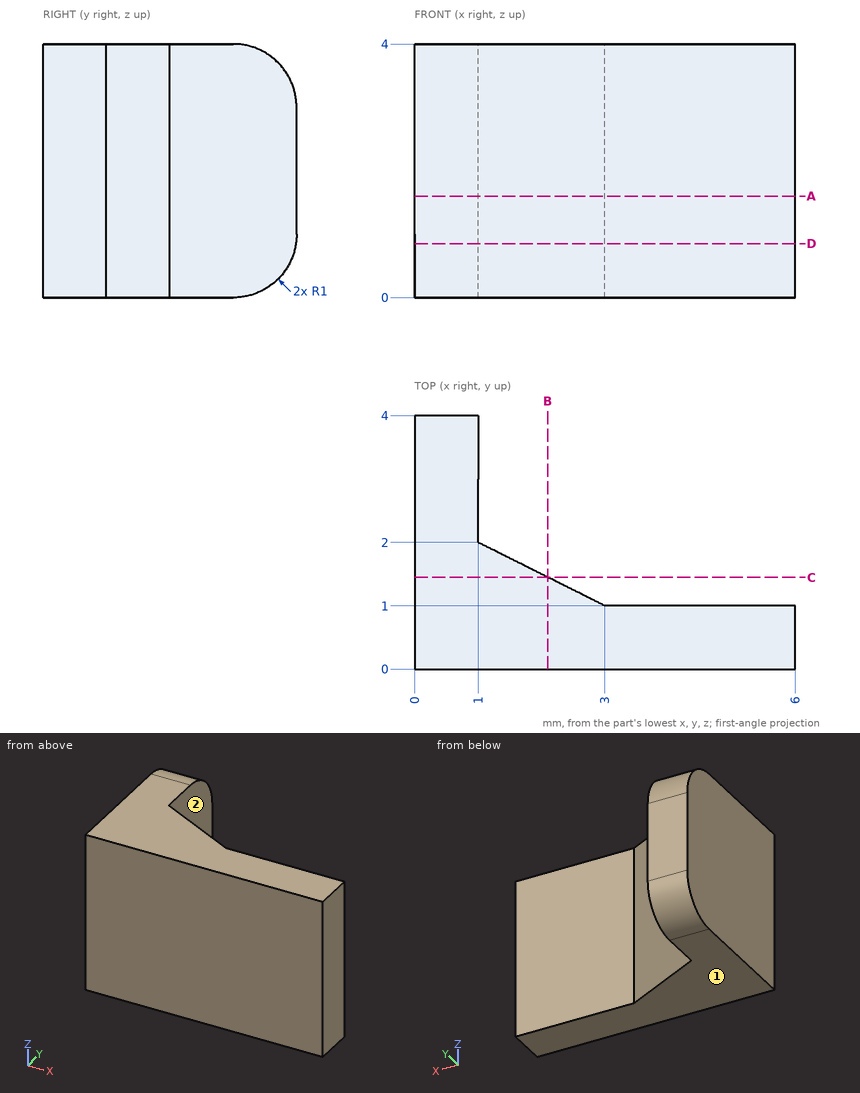
The drawing under review shows one solid part. Ordinate dimensions are in mm from its lowest x, y, z. A direction names the side the tool comes from. Round coordinates to 2 decimals unless told otherwise and drop trailing zeros. Write each loop counter-clockwise with the first axis right and the second up, starting at its lowest first coordinate (ties: lowest second). Pieces come first, ordered by that corner, then holes.
(1) We need section D-D on z = 0.85. Give the boundary of the cut face in (x, y), and give its area (3 significant figures).
(2) Insertion check: pin 1 (2 mm diameter, centred on y = 3.5, z = 3, fed in from +X); pin 2 (1.5 mm diameter, centred on y = 2, z = 2.5, fed in from +X). Each pin has a flat end and moves straight along its axis. Give the tip position at first contact, or say it passes through.
(3) We need section C-C on y = 1.45. Give the boundary of the cut face in (x, z).
(4) We need section A-A on z = 1.6. Give the boundary of the cut face in (x, y).
(5) Machinability: for the marked faces 1 and 2, which of the approach directions +Z, -Z, +X, -X, +Y, -Y give a long, thin tool a straight path to every point of the face, cutting with its end or side? Answer none if there is none.
(6) Wall thickness on L1, parallel to X at y = 3.65, z = 2.4; L2, parallel to X at y = 1.5, z = 2.65: over which ranges is each line inside the solid? List them lowest first.
(7) We need section B-B on x = 2.1. Give the boundary of the cut face in (y, z), and give its area (3 significant figures).
Findings below:
1. outline: (0, 0) - (6, 0) - (6, 1) - (3, 1) - (1, 2) - (1, 3.99) - (0, 3.99) - close
1. area: 9.99 mm2
2. pin 1: stops at x = 1
2. pin 2: stops at x = 2.5
3. outline: (0, 0) - (2.1, 0) - (2.1, 4) - (0, 4) - close
4. outline: (0, 0) - (6, 0) - (6, 1) - (3, 1) - (1, 2) - (1, 4) - (0, 4) - close
5. face 1: -Z, +X, -X, +Y, -Y
5. face 2: +Z, -Z, +X, +Y
6. L1: x = 0 to 1
6. L2: x = 0 to 2
7. outline: (0, 0) - (1.45, 0) - (1.45, 4) - (0, 4) - close
7. area: 5.80 mm2
